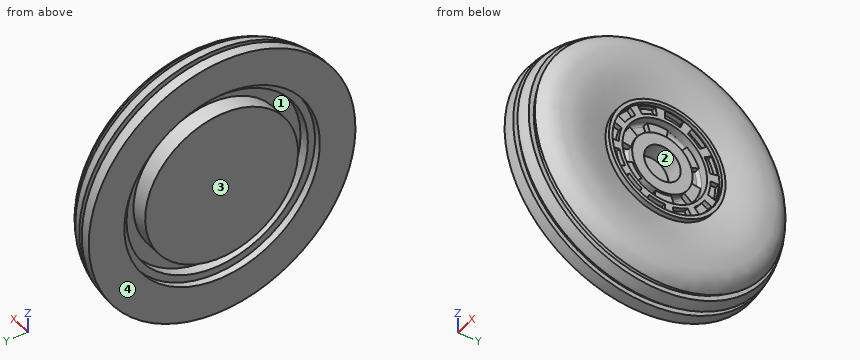
```python
from build123d import *

# Parameters (mm, degrees)
F2_W            = 0.2
F2_H            = 0.22
F3_ANGLE        = 20
F3_COPIES_COUNT = 12
F5_DEPTH        = 0.15


# Not quite as in the source:
# - a pattern or mirror of a feature is missing from the dataset's text; its kind, count and spacing are read off the source's solid


with BuildPart() as f1:
    # F0 (on Front) → F1 (revolve)
    with BuildSketch(Plane.XZ):
        with BuildLine():
            Line((1, 0.85), (0.87, 0.85))
            ThreePointArc((0.87, 0.85), (0.8134314575, 0.8734314575), (0.79, 0.93))
            Line((0.79, 0.93), (0.79, 1.11))
            ThreePointArc((0.79, 1.11), (0.8134314575, 1.1665685425), (0.87, 1.19))
            Line((0.87, 1.19), (1.1, 1.19))
            Line((1.1, 1.19), (1.1, 1.54))
            Line((1.1, 1.54), (1.2, 1.54))
            Line((1.2, 1.54), (1.2, 1.64))
            Line((1.2, 1.64), (1.12, 1.64))
            Line((1.12, 1.64), (1.0590550792, 1.64))
            add(Edge.make_bspline(
                [(1.0590550792, 1.64), (1.25, 2.3421209771), (1.2635455001, 2.685534462), (1.2259744013, 3.2558219262), (0.9930693577, 3.4693235058), (0.91, 3.5233867214)],
                knots=[0, 0, 0, 0, 0.3714125336, 0.6273384476, 0.7316891336, 0.7316891336, 0.7316891336, 0.7316891336], degree=3))
            Line((0.91, 3.5233867214), (0.91, 3.3833867214))
            Line((0.91, 3.3833867214), (0.77, 3.4602341654))
            Line((0.77, 3.4602341654), (0.77, 3.6002341654))
            add(Edge.make_bspline(
                [(0.77, 3.6002341654), (0.6784642229, 3.6425426702), (0.5744947558, 3.6771881754), (0.46, 3.7024604996)],
                knots=[0.7852748547, 0.7852748547, 0.7852748547, 0.7852748547, 0.8822719118, 0.8822719118, 0.8822719118, 0.8822719118], degree=3))
            Line((0.46, 3.7024604996), (0.46, 3.5624604996))
            Line((0.46, 3.5624604996), (0.32, 3.5878456739))
            Line((0.32, 3.5878456739), (0.32, 3.7278456739))
            add(Edge.make_bspline(
                [(0.32, 3.7278456739), (0.2195553432, 3.7423008552), (0.1125378698, 3.75), (0, 3.75)],
                knots=[0.9204576606, 0.9204576606, 0.9204576606, 0.9204576606, 1, 1, 1, 1], degree=3))
            Line((0, 3.75), (0, 2.75))
            Line((0, 2.75), (0.2, 2.75))
            Line((0.2, 2.75), (0.2, 2.55))
            Line((0.2, 2.55), (0.5, 2.55))
            Line((0.5, 2.55), (0.5, 2.15))
            Line((0.5, 2.15), (0.02, 2.15))
            Line((0.02, 2.15), (0.02, 0))
            Line((0.02, 0), (0.5, 0))
            Line((0.5, 0), (0.5, 0.515))
            Line((0.5, 0.515), (1, 0.515))
            Line((1, 0.515), (1, 0.85))
        make_face()
    revolve(axis=Axis((1.052, 0, 0), (1, 0, 0)))

    # F2 (on Front) → F3 (revolve, cut)
    with BuildSketch(Plane.XZ):
        with Locations((1.07, 1.4)):
            Rectangle(F2_W, F2_H)
    f3 = revolve(axis=Axis((1.36, 0, 0), (-1, 0, 0)), revolution_arc=F3_ANGLE, mode=Mode.SUBTRACT)

    # F3_copies: F3 ×12 about axis
    f3_copies_axis = Axis((0, 0, 0), (1, 0, 0))
    for i in range(1, F3_COPIES_COUNT):
        add(f3.rotate(f3_copies_axis, i * 360 / F3_COPIES_COUNT), mode=Mode.SUBTRACT)

    # F4 (on face) → F5 (join)
    with BuildSketch(Plane.YZ.offset(0.79)):
        with BuildLine():
            Line((-0.3895609432, 1.0703098951), (-0.2696546218, 0.7408699845))
            ThreePointArc((-0.2696546218, 0.7408699845), (-0.0687151015, 0.7854172037), (0.1369072395, 0.7764395384))
            Line((0.1369072395, 0.7764395384), (0.1977852744, 1.1216960307))
            ThreePointArc((0.1977852744, 1.1216960307), (-0.099270391, 1.1346657611), (-0.3895609432, 1.0703098951))
        make_face()
        with BuildLine():
            Line((-1.1216960307, 0.1977852744), (-0.7764395384, 0.1369072395))
            ThreePointArc((-0.7764395384, 0.1369072395), (-0.7145488017, 0.3331995784), (-0.603962745, 0.5067849166))
            Line((-0.603962745, 0.5067849166), (-0.8725246207, 0.7321350874))
            ThreePointArc((-0.8725246207, 0.7321350874), (-1.0322845694, 0.4813622001), (-1.1216960307, 0.1977852744))
        make_face()
        with BuildLine():
            Line((-0.7321350874, -0.8725246207), (-0.5067849166, -0.603962745))
            ThreePointArc((-0.5067849166, -0.603962745), (-0.6458337002, -0.4522176253), (-0.7408699845, -0.2696546218))
            Line((-0.7408699845, -0.2696546218), (-1.0703098951, -0.3895609432))
            ThreePointArc((-1.0703098951, -0.3895609432), (-0.9330141784, -0.653303561), (-0.7321350874, -0.8725246207))
        make_face()
        with BuildLine():
            Line((0.3895609432, -1.0703098951), (0.2696546218, -0.7408699845))
            ThreePointArc((0.2696546218, -0.7408699845), (0.0687151015, -0.7854172037), (-0.1369072395, -0.7764395384))
            Line((-0.1369072395, -0.7764395384), (-0.1977852744, -1.1216960307))
            ThreePointArc((-0.1977852744, -1.1216960307), (0.099270391, -1.1346657611), (0.3895609432, -1.0703098951))
        make_face()
        with BuildLine():
            Line((1.1216960307, -0.1977852744), (0.7764395384, -0.1369072395))
            ThreePointArc((0.7764395384, -0.1369072395), (0.7145488017, -0.3331995784), (0.603962745, -0.5067849166))
            Line((0.603962745, -0.5067849166), (0.8725246207, -0.7321350874))
            ThreePointArc((0.8725246207, -0.7321350874), (1.0322845694, -0.4813622001), (1.1216960307, -0.1977852744))
        make_face()
        with BuildLine():
            Line((0.7321350874, 0.8725246207), (0.5067849166, 0.603962745))
            ThreePointArc((0.5067849166, 0.603962745), (0.6458337002, 0.4522176253), (0.7408699845, 0.2696546218))
            Line((0.7408699845, 0.2696546218), (1.0703098951, 0.3895609432))
            ThreePointArc((1.0703098951, 0.3895609432), (0.9330141784, 0.653303561), (0.7321350874, 0.8725246207))
        make_face()
    extrude(amount=F5_DEPTH)


solid = f1.part
```
Design review of the part built by this model. Coordinates are the model's own, in mm. Face numbers are marked on the shaded views. A direction names the side the tool comes from. Round coordinates to 2 decimals unless told otherwise and drop trailing zeros.
Item 1: The part is to be moulded in two halves that separate along Z. For the marked faces 3 and 4, say which applies: +Z half, -Z half, draft (parallel to the pull), parting line (faces both ways), or undercut.
Item 2: For probe 1 along Y at (x, z) = (0.1, 0); probe 2 along Y at (x, z) = (0.15, 1.75), list the stretches that pass through material, from the lowest coordinate up.
Item 3: For the marked faces 1 and 2, list the 3-axis set-ups (+Z, -Z, +X, -X, +Y, -Y) from which the entire face can be reached by the end or side of a thin tool; tool diameter is ignored.
Item 4: Clearance check with flat-ended pins moving along their axes: pin 1 Ø0.5 at (y, z) = (1, 1) entering from +X; pin 2 Ø1.6 at (y, z) = (0, 0) entering from +X; pin 3 Ø1.6 at (y, z) = (0, -0.5) entering from -X. State where each tip first meets the part, or that it passes through.
Returned:
1. face 3: undercut
1. face 4: draft
2. probe 1: y = -3.75 to -2.75, -2.15 to 2.15, 2.75 to 3.75
2. probe 2: y = -3.31 to -2.12, -1.25 to 1.25, 2.12 to 3.31
3. face 1: -X
3. face 2: +X
4. pin 1: stops at x = 1.2
4. pin 2: stops at x = 1
4. pin 3: stops at x = 0.02
